Verification items for the finished model (mm, model axes). Face numbers are marked on the shaded views. A direction names the side the tool comes from. Give positions to 0.01 mm unless a question says otherwise; leave off trailing zeros. Write each loop counter-clockwise with the first axis right and the second up, starting at its lowest first coordinate (ties: lowest second). Pieces come first, ordered by that corner, then holes. Notation, with made-up numbers: (-36.5, 31) - (-27.5, 31) arc R34 ccw to (-27.5, 65) - close; hole circle Ø1 at (-26, 11). An arc over 180 degrees is marked (long way). Answer as a JSON object with one key per item and string values. Group by question number.
Item 1: Sectioned sample at D-D, the plane z = 3. Record the boundary of the cut face in (x, y).
Item 2: Sectioned sample at A-A, the plane y = 11.5. Record the boundary of the cut face in (x, z), and give its area (3 significant figures).
Item 3: Scan lines: line 1 along X through (y, z) = (8.89, -8.5); line 2 along Z through (x, y) = (26, 12); line 3 along X through (y, z) = (7.5, 7). Record each from-to range of solid material in increasing order. Write a range as [from, to].
Item 4: Sectioned sample at B-B, the plane y = 4.75. Record the boundary of the cut face in (x, z), and give its area (3 significant figures).
Item 5: Draft check along Y on the marked faces 1, 2 and 3. Enter one of: +Y half, -Y half, draft (parallel to the pull), parting line (faces both ways), or undercut.
Item 6: Go/stop test with a flat-tipped pin: pin 1 (2 mm diameter, centred on x = 29, z = 1, fed in from +Y). Record where the tip stops, or that it passes through.
Item 7: Sectioned sample at C-C, the plane x = 3. Record the boundary of the cut face in (y, z), and give its area (3 significant figures).
Item 8: Tool access check on the marked faces 4 and 5. Record the directions out of +Z, -Z, +X, -X, +Y, -Y that give a thin tool (end or side, any length) a straight path to the whole face; none if there is none.
```python
from build123d import *

# Parameters (mm, degrees)
SKETCH1_W                 = 76.2
SKETCH1_H                 = 34.925
BOSS_EXTRUDE1_DEPTH       = 12.7
SHELL1_T                  = -2.54
SHELL1_THICKNESS_2_FACE_W = 71.12
SHELL1_THICKNESS_2_FACE_H = 10.16
SHELL1_THICKNESS_2_DEPTH  = 1.27
SHELL1_THICKNESS_3_FACE_W = 71.12
SHELL1_THICKNESS_3_FACE_H = 10.16
SHELL1_THICKNESS_3_DEPTH  = 1.27
CUT_EXTRUDE4_DEPTH        = 28.575
CUT_EXTRUDE4_DEPTH_BACK   = 1.27
SKETCH10_W                = 76.2
SKETCH10_H                = 2.54
SKETCH11_W                = 2.54
SKETCH11_H                = 27.305
CUT_EXTRUDE5_DEPTH        = 2.54
FILL_START                = -10.141504854
FILL_PATTERN1_OUTLINE_R   = 1.143
FILL_PATTERN1_DEPTH       = 2.54
FILL_START_2              = 22.243495146
FILL_PATTERN2_OUTLINE_R   = 1.143
FILL_PATTERN2_DEPTH       = 2.54
SKETCH14_W                = 63.5
SKETCH14_H                = 5.08
BOSS_EXTRUDE2_DEPTH       = 0.762
SKETCH15_W                = 63.5
SKETCH15_H                = 5.08
BOSS_EXTRUDE3_DEPTH       = 0.762
SKETCH17_W                = 2.54
SKETCH17_H                = 19.685
BOSS_EXTRUDE4_DEPTH       = 5.08


# Read off the part's stored shape, not the designer's step: Fill Pattern1, Fill Pattern2
with BuildPart() as part:
    # Sketch1 → Boss-Extrude1 (new body)
    with BuildSketch(Plane(origin=(0, 0, 0), x_dir=(1, 0, 0), z_dir=(0, 1, 0))):
        with Locations((10.357281553, -7.320995146)):
            Rectangle(SKETCH1_W, SKETCH1_H)
    extrude(amount=BOSS_EXTRUDE1_DEPTH)

    # Shell1
    shell1_openings = [part.faces().sort_by_distance(p)[0] for p in [
        (10.357281553, 12.7, 7.320995146),
    ]]
    offset(amount=SHELL1_T, openings=shell1_openings, kind=Kind.INTERSECTION)

    # Shell1 thickness 2 face (on inner face of the shell) → Shell1 thickness 2 (add)
    with BuildSketch(Plane(origin=(10.357281553, 7.62, -7.601504854), x_dir=(-1, 0, 0), z_dir=(0, 0, -1))):
        Rectangle(SHELL1_THICKNESS_2_FACE_W, SHELL1_THICKNESS_2_FACE_H)
    extrude(amount=-SHELL1_THICKNESS_2_DEPTH)

    # Shell1 thickness 3 face (on inner face of the shell) → Shell1 thickness 3 (add)
    with BuildSketch(Plane(origin=(10.357281553, 7.62, 22.243495146), x_dir=(1, 0, 0), z_dir=(0, 0, 1))):
        Rectangle(SHELL1_THICKNESS_3_FACE_W, SHELL1_THICKNESS_3_FACE_H)
    extrude(amount=-SHELL1_THICKNESS_3_DEPTH)

    # Sketch10 → Cut-Extrude4 (cut, two sides: drawn at the far end of the back side and taken through both)
    with BuildSketch(Plane(origin=(0, 0, 20.973495146), x_dir=(-1, 0, 0), z_dir=(0, 0, -1)).offset(-CUT_EXTRUDE4_DEPTH_BACK)):
        with Locations((-10.357281553, 8.89)):
            Rectangle(SKETCH10_W, SKETCH10_H)
    extrude(amount=CUT_EXTRUDE4_DEPTH + CUT_EXTRUDE4_DEPTH_BACK, mode=Mode.SUBTRACT)

    # Sketch11 → Cut-Extrude5 (cut)
    with BuildSketch(Plane(origin=(0, 12.7, 0), x_dir=(1, 0, 0), z_dir=(0, 1, 0))):
        with Locations((-26.472718447, -7.320995146)):
            Rectangle(SKETCH11_W, SKETCH11_H)
        with Locations((47.187281553, -7.320995146)):
            Rectangle(SKETCH11_W, SKETCH11_H)
    extrude(amount=-CUT_EXTRUDE5_DEPTH, mode=Mode.SUBTRACT)

    # Fill Pattern1 outline → Fill Pattern1 (cut)
    with BuildSketch(Plane.XY.offset(FILL_START)):
        with Locations((10.357281553, 8.89)):
            Circle(FILL_PATTERN1_OUTLINE_R)
        with Locations((23.057281553, 8.89)):
            Circle(FILL_PATTERN1_OUTLINE_R)
        with Locations((35.757281553, 8.89)):
            Circle(FILL_PATTERN1_OUTLINE_R)
        with Locations((-2.342718447, 8.89)):
            Circle(FILL_PATTERN1_OUTLINE_R)
        with Locations((-15.042718447, 8.89)):
            Circle(FILL_PATTERN1_OUTLINE_R)
    extrude(amount=FILL_PATTERN1_DEPTH, mode=Mode.SUBTRACT)

    # Fill Pattern2 outline → Fill Pattern2 (cut)
    with BuildSketch(Plane.XY.offset(FILL_START_2)):
        with Locations((10.357281553, 8.89)):
            Circle(FILL_PATTERN2_OUTLINE_R)
        with Locations((23.057281553, 8.89)):
            Circle(FILL_PATTERN2_OUTLINE_R)
        with Locations((35.757281553, 8.89)):
            Circle(FILL_PATTERN2_OUTLINE_R)
        with Locations((-2.342718447, 8.89)):
            Circle(FILL_PATTERN2_OUTLINE_R)
        with Locations((-15.042718447, 8.89)):
            Circle(FILL_PATTERN2_OUTLINE_R)
    extrude(amount=FILL_PATTERN2_DEPTH, mode=Mode.SUBTRACT)

    # Sketch14 → Boss-Extrude2 (add)
    with BuildSketch(Plane.XY.offset(24.783495146)):
        with Locations((10.357281553, 8.89)):
            Rectangle(SKETCH14_W, SKETCH14_H)
    extrude(amount=-BOSS_EXTRUDE2_DEPTH)

    # Sketch15 → Boss-Extrude3 (add)
    with BuildSketch(Plane(origin=(0, 0, -10.141504854), x_dir=(-1, 0, 0), z_dir=(0, 0, -1))):
        with Locations((-10.357281553, 8.89)):
            Rectangle(SKETCH15_W, SKETCH15_H)
    extrude(amount=-BOSS_EXTRUDE3_DEPTH)

    # Sketch17 → Boss-Extrude4 (add)
    with BuildSketch(Plane(origin=(0, 7.62, 0), x_dir=(1, 0, 0), z_dir=(0, 1, 0))):
        with Locations((-26.472718447, -7.320995146)):
            Rectangle(SKETCH17_W, SKETCH17_H)
        with Locations((47.187281553, -7.320995146)):
            Rectangle(SKETCH17_W, SKETCH17_H)
    extrude(amount=BOSS_EXTRUDE4_DEPTH)


solid = part.part
```
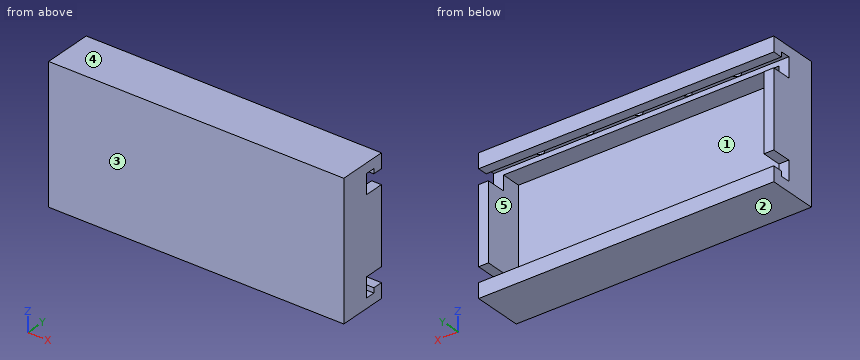
Geometry check:
{
 "1": {"outline": "(-27.74, 0) - (48.46, 0) - (48.46, 12.7) - (45.92, 12.7) - (45.92, 2.54) - (-25.2, 2.54) - (-25.2, 12.7) - (-27.74, 12.7) - close"},
 "2": {"outline": "(-27.74, -10.14) - (48.46, -10.14) - (48.46, -6.33) - (-27.74, -6.33) - close; (-27.74, -2.52) - (-25.2, -2.52) - (-25.2, 17.16) - (-27.74, 17.16) - close; (-27.74, 20.97) - (48.46, 20.97) - (48.46, 24.78) - (-27.74, 24.78) - close; (45.92, -2.52) - (48.46, -2.52) - (48.46, 17.16) - (45.92, 17.16) - close", "area": "681 mm^2"},
 "3": {"line 1": "[-27.74, -16.19], [-13.9, -3.49], [-1.2, 9.21], [11.5, 21.91], [24.2, 34.61], [36.9, 48.46]", "line 2": "[-10.14, -6.33], [20.97, 24.78]", "line 3": "[-27.74, -25.2], [45.92, 48.46]"},
 "4": {"outline": "(-27.74, -10.14) - (48.46, -10.14) - (48.46, 24.78) - (-27.74, 24.78) - close; hole (-25.2, -6.33) - (45.92, -6.33) - (45.92, 20.97) - (-25.2, 20.97) - close", "area": "719 mm^2"},
 "5": {"face 1": "+Y half", "face 2": "draft", "face 3": "-Y half"},
 "6": {"pin 1": "y = 2.54"},
 "7": {"outline": "(0, -10.14) - (12.7, -10.14) - (12.7, -6.33) - (10.16, -6.33) - (10.16, -7.6) - (7.62, -7.6) - (7.62, -6.33) - (2.54, -6.33) - (2.54, 20.97) - (7.62, 20.97) - (7.62, 22.24) - (10.16, 22.24) - (10.16, 20.97) - (12.7, 20.97) - (12.7, 24.78) - (0, 24.78) - close", "area": "160 mm^2"},
 "8": {"face 4": "+Z, +X, -X, +Y, -Y", "face 5": "+Y"}
}
